from build123d import *

# Parameters (mm, degrees)
F1_DEPTH = 355.6


with BuildPart() as f1:
    # F0 (on Right) → F1 (new body)
    with BuildSketch(Plane.YZ):
        Polygon((739.775, -9.525), (758.825, 9.525), (-758.825, 9.525), (-739.775, -9.525), (-384.175, -9.525), (-384.175, 0), (-365.125, 0), (-365.125, -9.525), (-9.525, -9.525), (-9.525, 0), (0, 0), (9.525, 0), (9.525, -9.525), (365.125, -9.525), (365.125, 0), (384.175, 0), (384.175, -9.525), align=None)
    extrude(amount=F1_DEPTH)


solid = f1.part
Design review of the part built by this model. Coordinates are the model's own, in mm. Round coordinates to 2 decimals unless told otherwise and drop trailing zeros. Order: outer loops, then holes, each group sorted by start corner. A loop starts at its lowest first (then second) coordinate and runs counter-clockwise, first axis right, second up. Notation, with made-up numbers: M -27.5,8.5 L 20.5,8.5 A25 ccw 20.5,39.5 Z; hole C 79,44.5 d5. An arc over 180 degrees is marked long. Answer as CSV lines item,"result". Start each with the question number.
1) Add section A-A (z = -3). Give the boundary of the cut face in (x, y) (3 decimals).
2) Add section B-B (x = 192). Give the boundary of the cut face in (y, z) (3 decimals), then the cut area to 3 significant figures.
3) Wall thickness on line 1 along Y through (x, z) = (152.5, -0.75) (3 decimals); line 2 along Y through (x, z) = (263, -7) (3 decimals); line 3 along Y through (x, z) = (314.5, 0.5): over which ranges is each line inside the solid? List them lowest first. Write a range as [from, to].
4) For pin 1 Ø3 at (x, z) = (159, -6) entering from +Y; pin 2 Ø7.5 at (x, z) = (218.5, -4) entering from -Y; pin 3 Ø6 at (x, z) = (156, -2) entering from -Y, all flat-tipped, find the tip position at first contact; note any pin that passes through.
Resolved:
1,outline,"M 0,-746.3 L 355.6,-746.3 L 355.6,-384.175 L 0,-384.175 Z; M 0,-365.125 L 355.6,-365.125 L 355.6,-9.525 L 0,-9.525 Z; M 0,9.525 L 355.6,9.525 L 355.6,365.125 L 0,365.125 Z; M 0,384.175 L 355.6,384.175 L 355.6,746.3 L 0,746.3 Z"
2,outline,"M -758.825,9.525 L -739.775,-9.525 L -384.175,-9.525 L -384.175,0 L -365.125,0 L -365.125,-9.525 L -9.525,-9.525 L -9.525,0 L 9.525,0 L 9.525,-9.525 L 365.125,-9.525 L 365.125,0 L 384.175,0 L 384.175,-9.525 L 739.775,-9.525 L 758.825,9.525 Z"
2,area,"28,000 mm^2"
3,line 1,"[-748.55, -384.175], [-365.125, -9.525], [9.525, 365.125], [384.175, 748.55]"
3,line 2,"[-742.3, -384.175], [-365.125, -9.525], [9.525, 365.125], [384.175, 742.3]"
3,line 3,"[-749.8, 749.8]"
4,pin 1,"y = 744.8"
4,pin 2,"y = -749.05"
4,pin 3,"y = -750.3"
